```python
from build123d import *

# Parameters (mm, degrees)
EXTRUDE_1_DEPTH     = 20
SKETCH_2_R          = 21
CUT_EXTRUDE_1_DEPTH = 31.812984276
SKETCH_3_R          = 1.6
CUT_EXTRUDE_2_DEPTH = 25.745908753
SKETCH_4_R          = 4
CUT_EXTRUDE_3_DEPTH = 25.007498873
FILLET_1_R          = 5
SKETCH_5_W          = 4
SKETCH_5_H          = 4
CUT_EXTRUDE_4_DEPTH = 25.745908796
SKETCH_6_R          = 4
CUT_EXTRUDE_5_DEPTH = 1


with BuildPart() as part:
    # 草图1 → 凸台-拉伸1 (new body)
    with BuildSketch(Plane(origin=(0, 0, 0), x_dir=(0, 0, -1), z_dir=(1, 0, 0))):
        Polygon((-10.6, 10), (10.6, 10), (10.6, -3), (7.6, -3), (7.6, 0), (-7.6, 0), (-7.6, -3), (-10.6, -3), align=None)
    extrude(amount=EXTRUDE_1_DEPTH)

    # 草图2 → 切除-拉伸1 (cut, through all)
    with BuildSketch(Plane.XY.offset(10.6)):
        with Locations((10, 30)):
            Circle(SKETCH_2_R)
    extrude(amount=-CUT_EXTRUDE_1_DEPTH, mode=Mode.SUBTRACT)

    # 草图3 → 切除-拉伸2 (cut, through all)
    with BuildSketch(Plane.XZ):
        with Locations(Location((10, 0, 0), (0, 0, 270))):
            Circle(SKETCH_3_R)
    extrude(amount=-CUT_EXTRUDE_2_DEPTH, mode=Mode.SUBTRACT)

    # 草图4 → 切除-拉伸3 (cut, through all)
    with BuildSketch(Plane(origin=(0, 5, 0), x_dir=(-1, 0, 0), z_dir=(0, -1, 0))):
        with Locations(Location((-10, 0, 0), (0, 0, 90))):
            Circle(SKETCH_4_R)
    extrude(amount=-CUT_EXTRUDE_3_DEPTH, mode=Mode.SUBTRACT)

    # 圆角1
    fillet_1_edges = [part.edges().sort_by_distance(p)[0] for p in [
        (16.403124237, 10, 0),
        (3.596875763, 10, 0),
    ]]
    fillet(fillet_1_edges, radius=FILLET_1_R)

    # 草图5 → 切除-拉伸4 (cut, through all)
    with BuildSketch(Plane(origin=(20, 0, 0), x_dir=(0, 0, -1), z_dir=(1, 0, 0))):
        with Locations((8.6, 8)):
            Rectangle(SKETCH_5_W, SKETCH_5_H)
    extrude(amount=-CUT_EXTRUDE_4_DEPTH, mode=Mode.SUBTRACT)

    # 草图6 → 切除-拉伸5 (cut)
    with BuildSketch(Plane.XZ):
        with Locations(Location((10, 0, 0), (0, 0, 270))):
            Circle(SKETCH_6_R)
    extrude(amount=-CUT_EXTRUDE_5_DEPTH, mode=Mode.SUBTRACT)


solid = part.part
```
Here's how the part is built. I have some questions about the finished solid (model axes, mm). A direction names the side the tool comes from. Round coordinates to 2 decimals unless told otherwise and drop trailing zeros. Order: outer loops, then holes, each group sorted by start corner. A loop starts at its lowest first (then second) coordinate and runs counter-clockwise, first axis right, second up. Notation, with made-up numbers: M -19.5,49 L -4.5,49 A23 ccw -4.5,77 Z; hole C 47,77 d11. An arc over 180 degrees is marked long. Answer in a Markdown table with one row per item.
Item 1: If I drill on L1, parallel to X at y = 0.6, z = 0; L2, parallel to X at y = 3, z = 0; L3, parallel to Z at x = 17.5, y = -1.5, over which ranges is the centre line in solid material (lowest first)? Write a range as from..to.
A:
| item | result |
|---|---|
| L1 | x = 0..6, 14..20 |
| L2 | x = 0..8.4, 11.6..20 |
| L3 | z = -10.6..-7.6, 7.6..10.6 |
Item 2: Imagine slicing it at D-D, the plane x = 4.5. Write out the boundary of the cut face in (y, z), and give its area (3 significant figures).
A:
| item | result |
|---|---|
| outline | M -3,-10.6 L 6,-10.6 L 6,-6.6 L 9.73,-6.6 L 9.73,10.6 L -3,10.6 L -3,7.6 L 0,7.6 L 0,-7.6 L -3,-7.6 Z |
| area | 209 mm2 |
Item 3: Thinking about a two-plate mould opening in X: for faces 1 (the face through (11.216, 9.035, 4.032)), 2 (the face through (10, -3, 9)), 3 (the face through (8, 5, 0)), 4 (the face through (0, 5, 0)), which applies, +X half, -X half, draft (parallel to the pull), parting line (faces both ways), or undercut?
A:
| item | result |
|---|---|
| face 1 | undercut |
| face 2 | draft |
| face 3 | undercut |
| face 4 | -X half |
Item 4: Imagine slicing it at A-A, the plane z = 0. Write out the boundary of the cut face in (x, y), and give its area (3 significant figures).
A:
| item | result |
|---|---|
| outline | M 0,0 L 6,0 L 6,1 L 8.4,1 L 8.4,5 L 6,5 L 6,9.38 A21 cw 4.23,9.81 A5 ccw 2.86,10 L 0,10 Z; M 11.6,1 L 14,1 L 14,0 L 20,0 L 20,10 L 17.14,10 A5 ccw 15.77,9.81 A21 cw 14,9.38 L 14,5 L 11.6,5 Z |
| area | 138 mm2 |
Item 5: Imagine slicing it at B-B, the plane x = 10. Write out the boundary of the cut face in (y, z), and give its area (3 significant figures).
A:
| item | result |
|---|---|
| outline | M -3,-10.6 L 6,-10.6 L 6,-6.6 L 9,-6.6 L 9,-4 L 5,-4 L 5,-1.6 L 1,-1.6 L 1,-4 L 0,-4 L 0,-7.6 L -3,-7.6 Z; M -3,7.6 L 0,7.6 L 0,4 L 1,4 L 1,1.6 L 5,1.6 L 5,4 L 9,4 L 9,10.6 L -3,10.6 Z |
| area | 144 mm2 |
Item 6: I'm going to push flat-ended pins straight in: pin 1 (9 mm diameter, centred on x = 10, z = 0, fed in from +Y); pin 2 (1.2 mm diameter, centred on x = 10.5, y = 8, fed in from -Z); pin 3 (6.5 mm diameter, centred on x = 8, z = 1.5, fed in from +Y); pin 4 (2 mm diameter, centred on y = 1, z = 6, fed in from -X). Where does each tip first touch, or does it pass through?
A:
| item | result |
|---|---|
| pin 1 | stops at y = 9.49 |
| pin 2 | stops at z = -6.6 |
| pin 3 | stops at y = 9.67 |
| pin 4 | stops at x = 0 |
Item 7: Imagine slicing it at C-C, the plane y = 2.75. Write out the boundary of the cut face in (x, z), and give its area (3 significant figures).
A:
| item | result |
|---|---|
| outline | M 0,-10.6 L 20,-10.6 L 20,10.6 L 0,10.6 Z; hole C 10,0 d3.2 |
| area | 416 mm2 |
Item 8: For faces 5 (the face through (7.6, 0, -3.5)), 6 (the face through (10, 8, -6.6)), 7 (the face through (16.44, 9.95, 2.12)), which set-ups out of +Z, -Z, +X, -X, +Y, -Y let a thin tool reach every point of the face, with its end or its side?
A:
| item | result |
|---|---|
| face 5 | +X, -X, -Y |
| face 6 | -Z, +X, -X, +Y |
| face 7 | +Z, -Z, +Y |
